from build123d import *

# Parameters (mm, degrees)
SKETCH1_R           = 21.2
SKETCH1_R_2         = 16.2
BOSS_EXTRUDE1_DEPTH = 20
FILLET1_R           = 1
SKETCH2_R           = 3
CUT_EXTRUDE1_DEPTH  = 10
CIRPATTERN1_COUNT   = 4


with BuildPart() as part:
    # Sketch1 → Boss-Extrude1 (new body)
    with BuildSketch(Plane(origin=(0, 0, 0), x_dir=(1, 0, 0), z_dir=(0, 1, 0))):
        with Locations(Location((0, 0, 0), (0, 0, 270))):
            Circle(SKETCH1_R)
        with Locations(Location((0, 0, 0), (0, 0, 270))):
            Circle(SKETCH1_R_2, mode=Mode.SUBTRACT)
    extrude(amount=BOSS_EXTRUDE1_DEPTH)

    # Fillet1
    fillet1_edges = [part.edges().sort_by_distance(p)[0] for p in [
        (0, 20, -16.2),
    ]]
    fillet(fillet1_edges, radius=FILLET1_R)

    # Sketch2 → Cut-Extrude1 (cut)
    with BuildSketch(Plane(origin=(21.2, 0, 0), x_dir=(0, 0, -1), z_dir=(1, 0, 0))):
        with Locations((0, 10)):
            Circle(SKETCH2_R)
    cut_extrude1 = extrude(amount=-CUT_EXTRUDE1_DEPTH, mode=Mode.SUBTRACT)

    # CirPattern1: Cut-Extrude1 ×4 about axis
    cirpattern1_axis = Axis((0, 19, 0), (0, -1, 0))
    for i in range(1, CIRPATTERN1_COUNT):
        add(cut_extrude1.rotate(cirpattern1_axis, i * 360 / CIRPATTERN1_COUNT), mode=Mode.SUBTRACT)


solid = part.part
Design review of the part built by this model. Coordinates are the model's own, in mm. Give positions to 0.01 mm unless a question says otherwise; leave off trailing zeros. Loops run counter-clockwise (first coordinate to the right, second up) from the corner with the lowest first, then second, coordinate; pieces in that order, holes last. Notation, with made-up numbers: M -9,58.25 L 27,58.25 A11 cw 27,66.25 Z; hole C 84.5,27 d11. An arc over 180 degrees is marked long. One line per question, with ' | ' between items. Start each with the question number.
1. Add section C-C (y = 10). Write out the cut boundary in (x, z).
2. Insertion check: P1, Ø4, axis at x = 15, y = 7.5, coming from the -Z side; P2, Ø2, axis at y = 9, z = 12, coming from the -X side; P3, Ø5, axis at x = -6, y = 15.5, coming from the +Z side. Each pin has a flat end and moves straight along its axis. Give the tip position at first contact, or say it passes through.
3. Add section B-B (z = 0). Write out the cut boundary in (x, y), plus the area to 3 significant figures.
4. The part is to be moulded in two halves that separate along X. For faces 1 (the face through (-8.12, 9.86, 19.583)), 2 (the face through (-2.86, 10.9, -18.6)), 3 (the face through (-18.59, 10.9, 2.86)), say which applies: released by +X, released by -X, zero draft, split by the parting line, or undercut.
5. Add section A-A (x = 0). Write out the cut boundary in (y, z).
6. To check wall thickness, follow L1, parallel to Y at x = 19, z = 0; L2, parallel to X at y = 13.5, z = 0; L3, parallel to Z at x = 15, y = 15. State the ranges of each line that lie inside material, in increasing order.
Worked out:
1) outline: M -20.99,-3 A21.2 ccw -3,-20.99 L -3,-15.92 A16.2 cw -15.92,-3 Z; M -20.99,3 L -15.92,3 A16.2 cw -3,15.92 L -3,20.99 A21.2 ccw Z; M 3,-20.99 A21.2 ccw 20.99,-3 L 15.92,-3 A16.2 cw 3,-15.92 Z; M 3,15.92 A16.2 cw 15.92,3 L 20.99,3 A21.2 ccw 3,20.99 Z
2) P1: stops at z = -16.75 | P2: stops at x = -18.12 | P3: stops at z = 20.91
3) outline: M -21.2,0 L -16.2,0 L -16.2,7 L -21.2,7 Z; M -21.2,13 L -16.2,13 L -16.2,19 A1 ccw -17.2,20 L -21.2,20 Z; M 16.2,0 L 21.2,0 L 21.2,7 L 16.2,7 Z; M 16.2,13 L 21.2,13 L 21.2,20 L 17.2,20 A1 ccw 16.2,19 Z | area: 140 mm²
4) face 1: split by the parting line | face 2: undercut | face 3: zero draft
5) outline: M 0,-21.2 L 7,-21.2 L 7,-16.2 L 0,-16.2 Z; M 0,16.2 L 7,16.2 L 7,21.2 L 0,21.2 Z; M 13,-21.2 L 20,-21.2 L 20,-17.2 A1 ccw 19,-16.2 L 13,-16.2 Z; M 13,16.2 L 19,16.2 A1 ccw 20,17.2 L 20,21.2 L 13,21.2 Z
6) L1: y = 0 to 7, 13 to 20 | L2: x = -21.2 to -16.2, 16.2 to 21.2 | L3: z = -14.98 to -6.12, 6.12 to 14.98
